Design review of the part built by this model. Coordinates are the model's own, in mm. Round coordinates to 2 decimals unless told otherwise and drop trailing zeros. Write each loop counter-clockwise with the first axis right and the second up, starting at its lowest first coordinate (ties: lowest second). Pieces come first, ordered by that corner, then holes. Notation, with made-up numbers: (78.25, 23.25) -> (135.25, 23.25) arc R30 cw to (135.25, 48.25) -> close; hole circle Ø3 at (71, -33.75). An arc over 180 degrees is marked (long way). Write item = value, one per line. Start each with the question number.
Item 1: Mouldability with a two-part tool opening along Z and no side actions: class faces 1 (the cylindrical face through (15.49, 1.52, -72.15)), 2 (the flat face through (0, 3, -1)), 3 (the cylindrical face through (1.83, 1.479, -32.493)) as released by +Z, released by -Z, zero draft, split by the parting line, or undercut.
Item 2: For pin 1 Ø12 at (x, z) = (1.5, -25) entering from -Y; pin 2 Ø5 at (x, z) = (-6, 62.5) entering from -Y, all flat-tipped, find the tip position at first contact; note any pin that passes through.
Item 3: Add section B-B, the plane x = 1.5. State the section outline as (y, z) points.
Item 4: Add section C-C, the plane y = 0.95. State the section outline as (x, z) points, then the cut area to 3 significant figures.
Item 5: Add section D-D, the plane z = -25. State the section outline as (x, y) points.
Item 6: Add section A-A, the plane z = 25. State the section outline as (x, y) points, then the cut area to 3 significant figures.
Item 7: To check wall thickness, follow L1, parallel to Z at x = 2, y = 2.45; L2, parallel to X at y = 1.9, z = -25; L3, parallel to X at y = 2.35, z = -62.5. State the ranges of each line that lie inside material, in increasing order.
from build123d import *

# Parameters (mm, degrees)
CROQUIS1_W              = 37
CROQUIS1_H              = 150
CROQUIS1_R              = 7.5
CROQUIS1_R_2            = 8.5
SALIENTE_EXTRUIR1_DEPTH = 3
REDONDEO1_R             = 10
CROQUIS2_R              = 2
CORTAR_EXTRUIR1_DEPTH   = 10


with BuildPart() as part:
    # Croquis1 → Saliente-Extruir1 (new body)
    with BuildSketch(Plane(origin=(0, 0, 0), x_dir=(1, 0, 0), z_dir=(0, 1, 0))):
        Rectangle(CROQUIS1_W, CROQUIS1_H)
        with Locations(Location((1.5, 25, 0), (0, 0, 270))):
            Circle(CROQUIS1_R, mode=Mode.SUBTRACT)
        with Locations(Location((1.5, -25, 0), (0, 0, 270))):
            Circle(CROQUIS1_R_2, mode=Mode.SUBTRACT)
    extrude(amount=SALIENTE_EXTRUIR1_DEPTH)

    # Redondeo1
    redondeo1_edges = [part.edges().sort_by_distance(p)[0] for p in [
        (18.5, 1.5, 75),
        (-18.5, 1.5, 75),
        (-18.5, 1.5, -75),
        (18.5, 1.5, -75),
    ]]
    fillet(redondeo1_edges, radius=REDONDEO1_R)

    # Croquis2 → Cortar-Extruir1 (cut)
    with BuildSketch(Plane(origin=(0, 3, 0), x_dir=(1, 0, 0), z_dir=(0, 1, 0))):
        with Locations(Location((-6, 62.5, 0), (0, 0, 270))):
            Circle(CROQUIS2_R)
        with Locations(Location((-6, -62.5, 0), (0, 0, 270))):
            Circle(CROQUIS2_R)
    extrude(amount=-CORTAR_EXTRUIR1_DEPTH, mode=Mode.SUBTRACT)


solid = part.part
Result set:
q1.face_1 = released by -Z
q1.face_2 = zero draft
q1.face_3 = undercut
q2.pin_1 = through
q2.pin_2 = 0
q3.outline = (0, -75) -> (3, -75) -> (3, -32.5) -> (0, -32.5) -> close; (0, -17.5) -> (3, -17.5) -> (3, 16.5) -> (0, 16.5) -> close; (0, 33.5) -> (3, 33.5) -> (3, 75) -> (0, 75) -> close
q4.outline = (-18.5, -65) arc R10 ccw to (-8.5, -75) -> (8.5, -75) arc R10 ccw to (18.5, -65) -> (18.5, 65) arc R10 ccw to (8.5, 75) -> (-8.5, 75) arc R10 ccw to (-18.5, 65) -> close; hole circle Ø4 at (-6, -62.5); hole circle Ø4 at (-6, 62.5); hole circle Ø17 at (1.5, 25); hole circle Ø15 at (1.5, -25)
q4.area = 5,040 mm²
q5.outline = (-18.5, 0) -> (-6, 0) -> (-6, 3) -> (-18.5, 3) -> close; (9, 0) -> (18.5, 0) -> (18.5, 3) -> (9, 3) -> close
q6.outline = (-18.5, 0) -> (-7, 0) -> (-7, 3) -> (-18.5, 3) -> close; (10, 0) -> (18.5, 0) -> (18.5, 3) -> (10, 3) -> close
q6.area = 60.0 mm²
q7.L1 = -75 to -32.48, -17.52 to 16.51, 33.49 to 75
q7.L2 = -18.5 to -6, 9 to 18.5
q7.L3 = -18.5 to -8, -4 to 18.5
